Check sheet for the drawn part. Datum: minimum x, y, z corner. Units: mm. Coordinates: 2 decimals unless noted, no trailing zeros. Loops run counter-clockwise (first coordinate to the right, second up) from the corner with the lowest first, then second, coordinate; pieces in that order, holes last. Notation, with made-up numbers: (-21.5, 1.25) - (11.5, 1.25) arc R25 cw to (11.5, 36.25) - close; hole circle Ø5 at (-13, 52.25). An arc over 180 degrees is marked (long way). Answer as a JSON object with one key per item and string values. Group by question number.
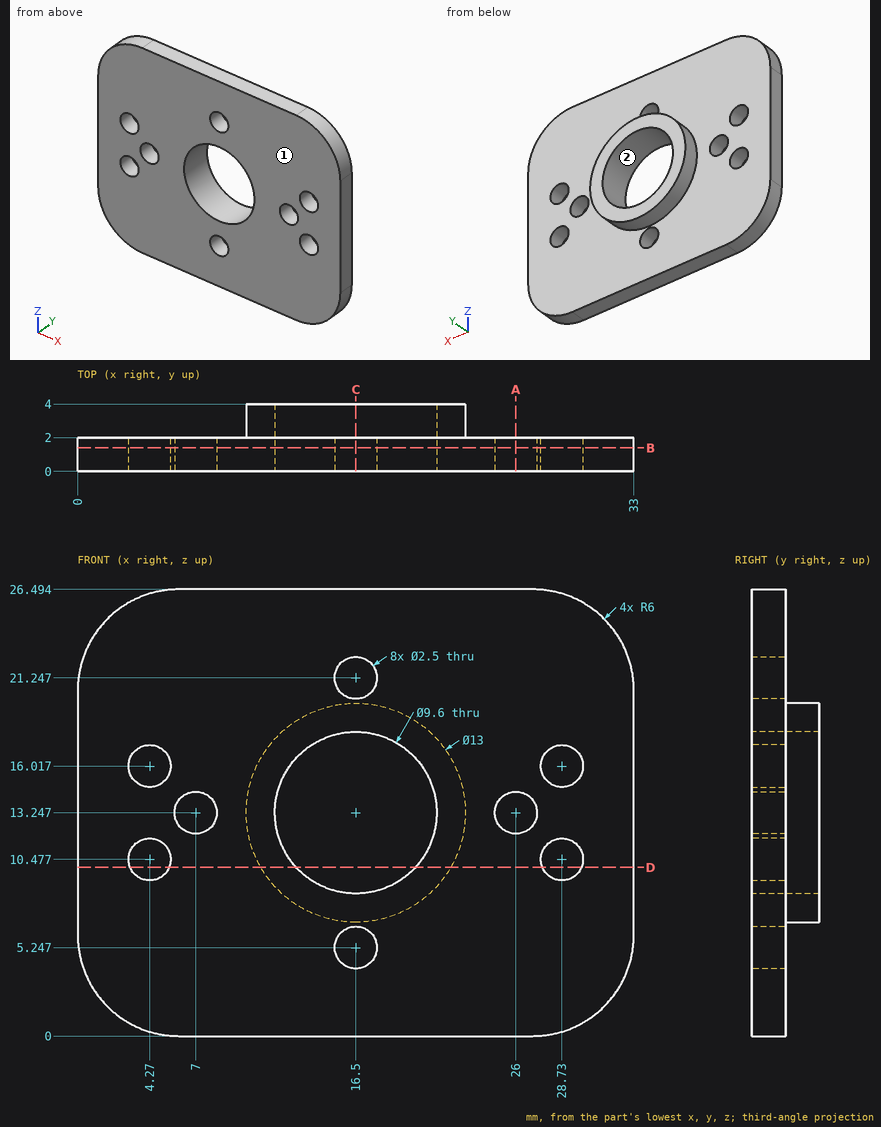
1. Gauge pin test, flat ends, axial feed: pin 1 (4 mm diameter, centred on x = 4.27, z = 10.48, fed in from +Y); pin 2 (1.5 mm diameter, centred on x = 28.73, z = 10.48, fed in from +Y); pin 3 (1.5 mm diameter, centred on x = 28, y = 0.5, fed in from -Z). Record the tip position at first contact, or that the pin passes through.
2. Sectioned sample at C-C on x = 16.5. Record the cut outline in (y, z), plus the area to 3 significant figures.
3. Release check for a two-part mould opening along X. For the marked faces 1 and 2 record: released by +X, released by -X, zero draft, split by the parting line, or undercut.
4. Sectioned sample at D-D on z = 10. Record the cut outline in (x, y) (1 decimal).
5. Material ranges on line 1 (Y direction, x = 9.5, z = 16); line 2 (X direction, y = 0.3, z = 12.5); line 3 (Z direction, x = 13, y = 0.85), recorded low to high.
6. Sectioned sample at A-A on x = 26. Record the cut outline in (y, z), plus the area to 3 significant figures.
7. Sectioned sample at B-B on y = 1.4. State how many separate pieces and enclosed holes the cut face has, plus the area to 3 significant figures.
Answers follow:
{
 "1": {"pin 1": "stops at y = 2", "pin 2": "passes through", "pin 3": "stops at z = 0.01"},
 "2": {"outline": "(0, 0) - (2, 0) - (2, 4) - (0, 4) - close; (0, 6.5) - (2, 6.5) - (2, 6.75) - (4, 6.75) - (4, 8.45) - (0, 8.45) - close; (0, 18.05) - (4, 18.05) - (4, 19.75) - (2, 19.75) - (2, 20) - (0, 20) - close; (0, 22.5) - (2, 22.5) - (2, 26.49) - (0, 26.49) - close", "area": "30.6 mm^2"},
 "3": {"face 1": "zero draft", "face 2": "undercut"},
 "4": {"outline": "(0, 0) - (3.1, 0) - (3.1, 2) - (0, 2) - close; (5.4, 0) - (13, 0) - (13, 4) - (10.9, 4) - (10.9, 2) - (5.4, 2) - close; (20, 0) - (27.6, 0) - (27.6, 2) - (22.1, 2) - (22.1, 4) - (20, 4) - close; (29.9, 0) - (33, 0) - (33, 2) - (29.9, 2) - close"},
 "5": {"line 1": "y = 0 to 2", "line 2": "x = 0 to 6, 8 to 11.76, 21.24 to 25, 27 to 33", "line 3": "z = 0 to 9.96, 16.53 to 26.49"},
 "6": {"outline": "(0, 0) - (2, 0) - (2, 12) - (0, 12) - close; (0, 14.5) - (2, 14.5) - (2, 26.49) - (0, 26.49) - close", "area": "48.0 mm^2"},
 "7": {"separate pieces": "1", "enclosed holes": "9", "area": "732 mm^2"}
}
